```python
from build123d import *

# Parameters (mm, degrees)
RESSALTO_EXTRUS_O1_DEPTH = 15
ESBO_O2_R                = 6
CORTE_EXTRUS_O1_DEPTH    = 185.458667457


with BuildPart() as part:
    # Esboço1 → Ressalto-extrusão1 (new body)
    with BuildSketch(Plane.XY):
        Polygon((0, 0), (130, 0), (82.683869545, 130), (47.316130455, 130), align=None)
    extrude(amount=RESSALTO_EXTRUS_O1_DEPTH)

    # Esboço2 → Corte-extrusão1 (cut, through all)
    with BuildSketch(Plane.XY.offset(15)):
        with Locations((65, 100)):
            Circle(ESBO_O2_R)
    extrude(amount=-CORTE_EXTRUS_O1_DEPTH, mode=Mode.SUBTRACT)


solid = part.part
```
Check sheet for the modelled part. Datum: model origin and axes. Units: mm. Round coordinates to 2 decimals unless told otherwise and drop trailing zeros. Order: outer loops, then holes, each group sorted by start corner. A loop starts at its lowest first (then second) coordinate and runs counter-clockwise, first axis right, second up.
1) Section check C-C (z = 8.5). Record the boundary of the cut face in (x, y), and give its area (3 significant figures).
2) Section check B-B (y = 95.5). Record the boundary of the cut face in (x, z).
3) Mould release check, pull along X, two halves, no side actions. Record for faces 1 (the flat face through (106.673, 64.09, 7.395)), 2 (the cylindrical face through (60.58, 104.06, 7.6)), 3 (the flat face through (64, 51, 0)): +X half, -X half, draft (parallel to the pull), parting line (faces both ways), or undercut.
4) Scan lines: line 1 (Y direction, x = 65, z = 7); line 2 (X direction, y = 46, z = 12.25); line 3 (X direction, y = 32, z = 12.25). Record each from-to range of solid material in increasing order.
5) Section check D-D (y = 36.5). Record the boundary of the cut face in (x, z), and give its area (3 significant figures).
6) Section check A-A (x = 65). Record the boundary of the cut face in (y, z).
7) Go/stop test with a flat-tipped pin: pin 1 Ø5 at (y, z) = (84.5, 13) entering from +X. Record where the tip stops, or that it passes through.
Result:
1. outline: (0, 0) - (130, 0) - (82.68, 130) - (47.32, 130) - close; hole circle Ø12 at (65, 100)
1. area: 10,600 mm2
2. outline: (34.76, 0) - (61.03, 0) - (61.03, 15) - (34.76, 15) - close; (68.97, 0) - (95.24, 0) - (95.24, 15) - (68.97, 15) - close
3. face 1: +X half
3. face 2: undercut
3. face 3: draft
4. line 1: y = 0 to 94, 106 to 130
4. line 2: x = 16.74 to 113.26
4. line 3: x = 11.65 to 118.35
5. outline: (13.28, 0) - (116.72, 0) - (116.72, 15) - (13.28, 15) - close
5. area: 1,550 mm2
6. outline: (0, 0) - (94, 0) - (94, 15) - (0, 15) - close; (106, 0) - (130, 0) - (130, 15) - (106, 15) - close
7. pin 1: stops at x = 100.15
